Here's how the part is built. I have some questions about the finished solid (model axes, mm). Face numbers are marked on the shaded views. A direction names the side the tool comes from. Round coordinates to 2 decimals unless told otherwise and drop trailing zeros. Write each loop counter-clockwise with the first axis right and the second up, starting at its lowest first coordinate (ties: lowest second). Pieces come first, ordered by that corner, then holes. Notation, with made-up numbers: M -8,12 L 31,12 A18 ccw 31,30 Z; hole C 58.5,74 d1. An arc over 180 degrees is marked long. Write item = value, one per line. Start each with the question number.
(1) I want a section at B-B (x = 17.5). List the corners of the cut face in (y, z) for me, and give its area (3 significant figures).
(2) If we mould it in two halves opening along Y, with no side actions, what happens to the marked faces 1, 2 and 3? For each: released by +Y, released by -Y, zero draft, split by the parting line, or undercut.
(3) Will these pins go through, and if not, where does the flat tip stop? pin 1 Ø1 at (y, z) = (2, 7.5) entering from +X; pin 2 Ø3 at (x, z) = (-16, 4.5) entering from -Y; pin 3 Ø2.5 at (y, z) = (-8.5, 2.5) entering from -X.
(4) I want a section at D-D (y = 5). List the corners of the cut face in (x, z) for me, and give its area (3 significant figures).
(5) On a 3-axis mill with a long thin cutter (end or side, diameter ignored), from which of +Z, -Z, +X, -X, +Y, -Y can I reach the whole of each face in a straight line? I mean the marked faces 4, 5, 6 and 7. Say none if no direction works.
(6) I want a section at C-C (x = -13.5). List the corners of the cut face in (y, z) for me.
(7) I want a section at A-A (z = 12.25). List the corners of the cut face in (x, y) for me (3 decimals), and give its area (3 significant figures).
(8) I need wall thicknesses on line 1 along Y through (x, z) = (18.5, 1); line 2 along Z through (x, y) = (-8, -5.5); line 3 along Z through (x, y) = (2, -8.75). Which ranges of each line are inside material? Lowest first, please.
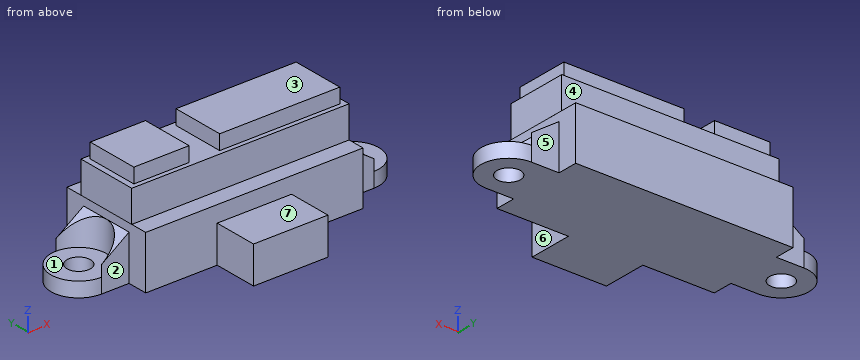
```python
from build123d import *

# Parameters (mm, degrees)
SKETCH1_W           = 29.5
SKETCH1_H           = 13
BOSS_EXTRUDE1_DEPTH = 7.2
BOSS_EXTRUDE2_DEPTH = 4.3
SKETCH3_W           = 7.5
SKETCH3_H           = 7.2
SKETCH3_W_2         = 16.3
BOSS_EXTRUDE3_DEPTH = 2
SKETCH4_R           = 1.6
BOSS_EXTRUDE6_DEPTH = 2
SKETCH6_W           = 10.1
SKETCH6_H           = 6
BOSS_EXTRUDE7_DEPTH = 5
SKETCH7_W           = 3.75
SKETCH7_H           = 7.5
BOSS_EXTRUDE8_DEPTH = 4.1
CUT_EXTRUDE1_START  = -4.1
SKETCH8_R           = 3.75
CUT_EXTRUDE1_DEPTH  = 4.1
CUT_EXTRUDE2_DEPTH  = 31.681835017


with BuildPart() as part:
    # Sketch1 → Boss-Extrude1 (new body)
    with BuildSketch(Plane.XY):
        Rectangle(SKETCH1_W, SKETCH1_H)
    extrude(amount=BOSS_EXTRUDE1_DEPTH)

    # Sketch2 → Boss-Extrude2 (add)
    with BuildSketch(Plane.XY.offset(7.2)):
        Polygon((-14.746484108, 4.199496061), (14.753515892, 4.199496061), (14.75, -4.200497315), (-14.757033461, -4.200497315), align=None)
    extrude(amount=BOSS_EXTRUDE2_DEPTH)

    # Sketch3 → Boss-Extrude3 (add)
    with BuildSketch(Plane.XY.offset(11.5)):
        with Locations((-10.225, 0)):
            Rectangle(SKETCH3_W, SKETCH3_H)
        with Locations((5.825, 0)):
            Rectangle(SKETCH3_W_2, SKETCH3_H)
    extrude(amount=BOSS_EXTRUDE3_DEPTH)

    # Sketch4 → Boss-Extrude6 (add)
    # profile 1 of 2: a face of its own
    with BuildSketch(Plane(origin=(0, 0, 0), x_dir=(-1, 0, 0), z_dir=(0, 0, -1))):
        with BuildLine():
            Line((-14.75, 3.75), (-14.75, -3.75))
            Line((-14.75, -3.75), (-18.5, -3.75))
            ThreePointArc((-18.5, -3.75), (-22.25, 0), (-18.5, 3.75))
            Line((-18.5, 3.75), (-14.75, 3.75))
        make_face()
        with Locations(Location((-18.5, 0, 0), (0, 0, 180))):
            Circle(SKETCH4_R, mode=Mode.SUBTRACT)
    # profile 2 of 2: a face of its own
    with BuildSketch(Plane(origin=(0, 0, 0), x_dir=(-1, 0, 0), z_dir=(0, 0, -1))):
        with BuildLine():
            Line((18.5, 3.75), (14.75, 3.75))
            Line((14.75, 3.75), (14.75, -3.75))
            Line((14.75, -3.75), (18.5, -3.75))
            ThreePointArc((18.5, -3.75), (22.25, 0), (18.5, 3.75))
        make_face()
        with Locations((18.5, 0)):
            Circle(SKETCH4_R, mode=Mode.SUBTRACT)
    extrude(amount=-BOSS_EXTRUDE6_DEPTH)

    # Sketch6 → Boss-Extrude7 (add)
    with BuildSketch(Plane(origin=(0, 0, 0), x_dir=(-1, 0, 0), z_dir=(0, 0, -1))):
        with Locations((0, -9.5)):
            Rectangle(SKETCH6_W, SKETCH6_H)
    extrude(amount=-BOSS_EXTRUDE7_DEPTH)

    # Sketch7 → Boss-Extrude8 (add)
    with BuildSketch(Plane.XY.offset(2)):
        with Locations((-16.625, 0)):
            Rectangle(SKETCH7_W, SKETCH7_H)
        with Locations((16.625, 0)):
            Rectangle(SKETCH7_W, SKETCH7_H)
    extrude(amount=BOSS_EXTRUDE8_DEPTH)

    # Sketch8 → Cut-Extrude1 (cut)
    with BuildSketch(Plane.XY.offset(6.1).offset(CUT_EXTRUDE1_START)):
        with Locations((-18.5, 0)):
            Circle(SKETCH8_R)
        with Locations((18.5, 0)):
            Circle(SKETCH8_R)
    extrude(amount=CUT_EXTRUDE1_DEPTH, mode=Mode.SUBTRACT)

    # Sketch9 → Cut-Extrude2 (cut, through all)
    with BuildSketch(Plane(origin=(0, 3.75, 0), x_dir=(1, 0, 0), z_dir=(0, 1, 0))):
        Polygon((-18.5, -3.5), (-14.75, -6.1), (-18.5, -6.1), align=None)
        Polygon((18.5, -6.1), (18.5, -3.5), (14.75, -6.1), align=None)
    extrude(amount=-CUT_EXTRUDE2_DEPTH, mode=Mode.SUBTRACT)


solid = part.part
```
Returned:
q1.outline = M -3.75,0 L -1.25,0 L -1.25,2 L -3.61,2 L -3.61,4.19 L -3.75,4.19 Z; M 1.25,0 L 3.75,0 L 3.75,4.19 L 3.61,4.19 L 3.61,2 L 1.25,2 Z
q1.area = 10.6 mm²
q2.face_1 = undercut
q2.face_2 = released by -Y
q2.face_3 = zero draft
q3.pin_1 = 14.75
q3.pin_2 = -6.5
q3.pin_3 = -5.05
q4.outline = M -14.75,0 L 14.75,0 L 14.75,7.2 L -14.75,7.2 Z
q4.area = 212 mm²
q5.face_4 = +Z, +X, -X, +Y
q5.face_5 = +Z, -Z, +X, +Y
q5.face_6 = +Z, -Z, +X, -Y
q5.face_7 = +Z, +X, -X, -Y
q6.outline = M -6.5,0 L 6.5,0 L 6.5,7.2 L 4.2,7.2 L 4.2,11.5 L 3.6,11.5 L 3.6,13.5 L -3.6,13.5 L -3.6,11.5 L -4.2,11.5 L -4.2,7.2 L -6.5,7.2 Z
q7.outline = M -13.975,-3.6 L -6.475,-3.6 L -6.475,3.6 L -13.975,3.6 Z; M -2.325,-3.6 L 13.975,-3.6 L 13.975,3.6 L -2.325,3.6 Z
q7.area = 171 mm²
q8.line_1 = -3.75 to -1.6, 1.6 to 3.75
q8.line_2 = 0 to 7.2
q8.line_3 = 0 to 5
